Can you work these out from the model? Positions are in its coordinate system, mm. A direction names the side the tool comes from. Round coordinates to 2 decimals unless told otherwise and drop trailing zeros. Loops run counter-clockwise (first coordinate to the right, second up) from the corner with the lowest first, then second, coordinate; pieces in that order, holes last. Notation, with made-up numbers: (-13.5, 73.25) -> (13.5, 73.25) arc R16 cw to (13.5, 78.25) -> close; hole circle Ø1 at (-38.5, -1.75). An arc over 180 degrees is marked (long way). Use a Markdown table: item, result.
from build123d import *

# Parameters (mm, degrees)
SKETCH1_W           = 20
SKETCH1_H           = 20
SKETCH1_W_2         = 18
SKETCH1_H_2         = 18
BOSS_EXTRUDE1_DEPTH = 80
SKETCH2_R           = 2.25
CUT_EXTRUDE1_DEPTH  = 84.066238629
SKETCH3_R           = 2.25
CUT_EXTRUDE2_DEPTH  = 84.066238629


with BuildPart() as part:
    # Sketch1 → Boss-Extrude1 (new body)
    with BuildSketch(Plane(origin=(0, 0, 0), x_dir=(1, 0, 0), z_dir=(0, 1, 0))):
        Rectangle(SKETCH1_W, SKETCH1_H)
        Rectangle(SKETCH1_W_2, SKETCH1_H_2, mode=Mode.SUBTRACT)
    extrude(amount=BOSS_EXTRUDE1_DEPTH)

    # Sketch2 → Cut-Extrude1 (cut, through all)
    with BuildSketch(Plane.XY.offset(10)):
        with Locations((0, 10)):
            Circle(SKETCH2_R)
        with Locations((0, 30)):
            Circle(SKETCH2_R)
    extrude(amount=-CUT_EXTRUDE1_DEPTH, mode=Mode.SUBTRACT)

    # Sketch3 → Cut-Extrude2 (cut, through all)
    with BuildSketch(Plane(origin=(10, 0, 0), x_dir=(0, 0, -1), z_dir=(1, 0, 0))):
        with Locations((0, 70)):
            Circle(SKETCH3_R)
    extrude(amount=-CUT_EXTRUDE2_DEPTH, mode=Mode.SUBTRACT)


solid = part.part
1. Will this pin go through, and if not, where does the flat tip stop? pin 1 Ø7 at (x, y) = (0, 30) entering from -Z.
Answer sheet:
| item | result |
|---|---|
| pin 1 | stops at z = -10 |
2. I want a section at C-C (x = -5.5). Please give me the cut outline in (y, z), plus the area to 3 significant figures.
Answer sheet:
| item | result |
|---|---|
| outline | (0, -10) -> (80, -10) -> (80, -9) -> (0, -9) -> close; (0, 9) -> (80, 9) -> (80, 10) -> (0, 10) -> close |
| area | 160 mm² |
3. I need wall thicknesses on line 1 (Y direction, x = 0, z = 9.65); line 2 (X direction, y = 47, z = -1). Which ranges of each line are inside material? Lowest first, please.
Answer sheet:
| item | result |
|---|---|
| line 1 | y = 0 to 7.75, 12.25 to 27.75, 32.25 to 80 |
| line 2 | x = -10 to -9, 9 to 10 |
4. Which directions (+Z, -Z, +X, -X, +Y, -Y) give clear straight access to the entire face, cutting with the end or side of a thin tool? Please do faces 1 (the flat face through (-10, 39, 0)), 2 (the flat face through (9, 39, 0)).
Answer sheet:
| item | result |
|---|---|
| face 1 | +Z, -Z, -X, +Y, -Y |
| face 2 | +Y, -Y |
5. I want a section at A-A (z = 5.25). Please give me the cut outline in (x, y), plus the area to 3 significant figures.
Answer sheet:
| item | result |
|---|---|
| outline | (-10, 0) -> (-9, 0) -> (-9, 80) -> (-10, 80) -> close; (9, 0) -> (10, 0) -> (10, 80) -> (9, 80) -> close |
| area | 160 mm² |
6. If we mould it in two halves opening along Z, with no side actions, what happens to faces 3 (the flat face through (0, 39, -10)), 4 (the cylindrical face through (-0.488, 27.804, -9.493)), 5 (the cylindrical face through (-9.493, 67.804, 0.488))? For each: +Z half, -Z half, draft (parallel to the pull), parting line (faces both ways), or undercut.
Answer sheet:
| item | result |
|---|---|
| face 3 | -Z half |
| face 4 | draft |
| face 5 | undercut |
7. I want a section at B-B (y = 13.5). Please give me the cut outline in (x, z).
Answer sheet:
| item | result |
|---|---|
| outline | (-10, -10) -> (10, -10) -> (10, 10) -> (-10, 10) -> close; hole (-9, -9) -> (9, -9) -> (9, 9) -> (-9, 9) -> close |
8. I want a section at D-D (z = 0). Please give me the cut outline in (x, y), plus the area to 3 significant figures.
Answer sheet:
| item | result |
|---|---|
| outline | (-10, 0) -> (-9, 0) -> (-9, 67.75) -> (-10, 67.75) -> close; (-10, 72.25) -> (-9, 72.25) -> (-9, 80) -> (-10, 80) -> close; (9, 0) -> (10, 0) -> (10, 67.75) -> (9, 67.75) -> close; (9, 72.25) -> (10, 72.25) -> (10, 80) -> (9, 80) -> close |
| area | 151 mm² |
